Work out the finished part from the listing and answer in its coordinate system (mm). A direction names the side the tool comes from. Give positions to 0.01 mm unless a question says otherwise; leave off trailing zeros. Order: outer loops, then holes, each group sorted by start corner. A loop starts at its lowest first (then second) coordinate and runs counter-clockwise, first axis right, second up. Notation, with made-up numbers: (70, 50) -> (95, 50) arc R18 ccw to (95, 81) -> close; hole circle Ø3 at (43.25, 38.5). An arc over 180 degrees is marked (long way). Use a Markdown table: item, result. Add a question column.
```python
from build123d import *

# Parameters (mm, degrees)
SKETCH_1_W          = 95.7
SKETCH_1_H          = 95.7
SKETCH_1_W_2        = 85.7
SKETCH_1_H_2        = 85.7
EXTRUDE_1_DEPTH     = 8.6
SKETCH_2_W          = 8.6
SKETCH_2_H          = 95.7
EXTRUDE_2_DEPTH     = 25
CUT_EXTRUDE_2_DEPTH = 90.7


with BuildPart() as part:
    # 草图1 → 凸台-拉伸1 (new body)
    with BuildSketch(Plane.XY):
        Rectangle(SKETCH_1_W, SKETCH_1_H)
        Rectangle(SKETCH_1_W_2, SKETCH_1_H_2, mode=Mode.SUBTRACT)
    extrude(amount=EXTRUDE_1_DEPTH)

    # 草图2 → 凸台-拉伸2 (add)
    with BuildSketch(Plane.ZY.offset(47.85)):
        with Locations((4.3, 0)):
            Rectangle(SKETCH_2_W, SKETCH_2_H)
    extrude(amount=EXTRUDE_2_DEPTH)

    # 草图5 → 切除-拉伸2 (cut)
    with BuildSketch(Plane(origin=(0, 47.85, 0), x_dir=(1, 0, 0), z_dir=(0, 1, 0))):
        Polygon((-67.35, -8.6), (-63.35, -8.6), (-63.35, -5.6), (-61.85, -5.6), (-61.85, -3.1), (-68.85, -3.1), (-68.85, -5.6), (-67.35, -5.6), align=None)
        Polygon((-53.85, -5.6), (-53.85, -3.1), (-46.85, -3.1), (-46.85, -5.6), (-48.35, -5.6), (-48.35, -8.6), (-52.35, -8.6), (-52.35, -5.6), align=None)
    extrude(amount=-CUT_EXTRUDE_2_DEPTH, mode=Mode.SUBTRACT)


solid = part.part
```
1) Straight lines are drawn through the part: line 1 (X direction, y = -14, z = 7.75); line 2 (X direction, y = -13, z = 4.25); line 3 (X direction, y = 43.5, z = 7.5). For each, find the intervals that lie inside material, in ascending order.
2) Determine the mould class of faces 4 (the flat face through (-46.85, 3, 4)), 5 (the flat face through (-12, -47.85, 4)), 6 (the flat face through (-72.85, 1, 4)) for opening direction X: released by +X, released by -X, zero draft, split by the parting line, or undercut.
3) The part is cut by section B-B, the plane z = 7. Determine the outline of the cut face in (x, y), then the cut area to 3 significant figures.
4) Which of the six approach directions +Z, -Z, +X, -X, +Y, -Y give full straight-line access (tool end or side, diameter ignored) to faces 1 (the flat face through (-48.35, 3, 7)), 2 (the flat face through (-1, 42.85, 4)), 3 (the flat face through (-65, 3, 3.1))?
5) The part is cut by section A-A, the plane x = -31. Determine the outline of the cut face in (y, z), then the cut area to 3 significant figures.
6) The part is cut by section C-C, the plane y = -20.5. Determine the outline of the cut face in (x, z).
7) A flat-ended cylindrical pin translates along its axis: pin 1 (4.5 mm diameter, centred on x = -65.5, z = 5.5, fed in from +Y). Find the tip coordinate at first contact, or state that the pin passes through.
A:
| question | item | result |
|---|---|---|
| 1 | line 1 | -72.85 to -67.35, -63.35 to -52.35, -48.35 to -42.85, 42.85 to 47.85 |
| 1 | line 2 | -72.85 to -68.85, -61.85 to -53.85, -46.85 to -42.85, 42.85 to 47.85 |
| 1 | line 3 | -72.85 to -67.35, -63.35 to -52.35, -48.35 to 47.85 |
| 2 | face 4 | undercut |
| 2 | face 5 | zero draft |
| 2 | face 6 | released by -X |
| 3 | outline | (-72.85, -47.85) -> (47.85, -47.85) -> (47.85, 47.85) -> (-48.35, 47.85) -> (-48.35, -42.85) -> (-52.35, -42.85) -> (-52.35, 47.85) -> (-63.35, 47.85) -> (-63.35, -42.85) -> (-67.35, -42.85) -> (-67.35, 47.85) -> (-72.85, 47.85) -> close; hole (-42.85, -42.85) -> (42.85, -42.85) -> (42.85, 42.85) -> (-42.85, 42.85) -> close |
| 3 | area | 3,480 mm^2 |
| 4 | face 1 | +Z, +Y |
| 4 | face 2 | +Z, -Z |
| 4 | face 3 | +Y |
| 5 | outline | (-47.85, 0) -> (-42.85, 0) -> (-42.85, 8.6) -> (-47.85, 8.6) -> close; (42.85, 0) -> (47.85, 0) -> (47.85, 8.6) -> (42.85, 8.6) -> close |
| 5 | area | 86.0 mm^2 |
| 6 | outline | (-72.85, 0) -> (-42.85, 0) -> (-42.85, 8.6) -> (-48.35, 8.6) -> (-48.35, 5.6) -> (-46.85, 5.6) -> (-46.85, 3.1) -> (-53.85, 3.1) -> (-53.85, 5.6) -> (-52.35, 5.6) -> (-52.35, 8.6) -> (-63.35, 8.6) -> (-63.35, 5.6) -> (-61.85, 5.6) -> (-61.85, 3.1) -> (-68.85, 3.1) -> (-68.85, 5.6) -> (-67.35, 5.6) -> (-67.35, 8.6) -> (-72.85, 8.6) -> close; (42.85, 0) -> (47.85, 0) -> (47.85, 8.6) -> (42.85, 8.6) -> close |
| 7 | pin 1 | y = 47.85 |
